from build123d import *

# Parameters (mm, degrees)
CROQUIS1_R              = 20
CROQUIS1_R_2            = 1.5
SALIENTE_EXTRUIR1_DEPTH = 2
CROQUIS2_R              = 5.75
CORTAR_EXTRUIR1_DEPTH   = 10


with BuildPart() as part:
    # Croquis1 → Saliente-Extruir1 (new body)
    with BuildSketch(Plane.XY):
        Circle(CROQUIS1_R)
        with Locations((15, 8.1)):
            Circle(CROQUIS1_R_2, mode=Mode.SUBTRACT)
        with Locations((0, -16)):
            Circle(CROQUIS1_R_2, mode=Mode.SUBTRACT)
        with Locations(Location((-15, 8.1, 0), (0, 0, 180))):
            Circle(CROQUIS1_R_2, mode=Mode.SUBTRACT)
    extrude(amount=SALIENTE_EXTRUIR1_DEPTH)

    # Croquis2 → Cortar-Extruir1 (cut)
    with BuildSketch(Plane.XY.offset(2)):
        Circle(CROQUIS2_R)
    extrude(amount=-CORTAR_EXTRUIR1_DEPTH, mode=Mode.SUBTRACT)


solid = part.part
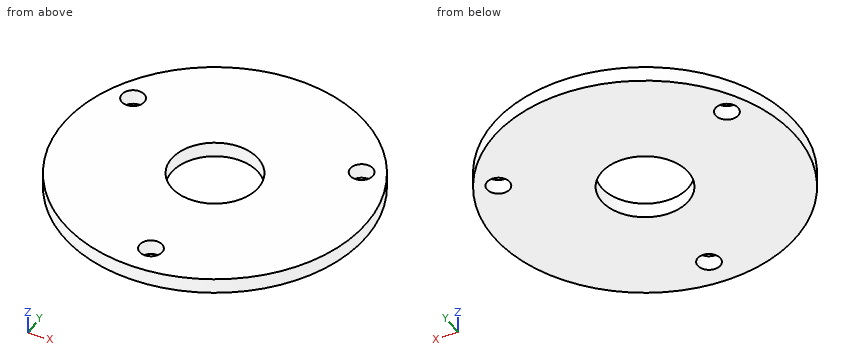
Design review of the part built by this model. Coordinates are the model's own, in mm. Coordinates: 2 decimals unless noted, no trailing zeros. Order: outer loops, then holes, each group sorted by start corner. A loop starts at its lowest first (then second) coordinate and runs counter-clockwise, first axis right, second up. Notation, with made-up numbers: (5, -4.75) - (55, -4.75) arc R20 cw to (55, 21.25) - close; hole circle Ø11 at (25, -39.5). An arc over 180 degrees is marked (long way). Put each result on its own line as item: value.
1) Take a section at D-D, the plane x = 12. Give the boundary of the cut face in (y, z).
Response values:
outline: (-16, 0) - (16, 0) - (16, 2) - (-16, 2) - close
2) Insertion check: P1, Ø13, axis at x = 0, y = 0, coming from the -Z side; P2, Ø1, axis at x = 7.5, z = 0.5, coming from the -Y side (3 decimals); P3, Ø1, axis at y = 12, z = 0.5, coming from the -X side; P4, Ø1, axis at y = -4, z = 0.5, coming from the -X side. Each pin has a flat end and moves straight along its axis. Give the tip position at first contact, or say it passes through.
Response values:
P1: stops at z = 0
P2: stops at y = -18.735
P3: stops at x = -16.36
P4: stops at x = -19.69
3) Take a section at A-A, the plane y = -16. Give the boundary of the cut face in (x, z).
Response values:
outline: (-12, 0) - (-1.5, 0) - (-1.5, 2) - (-12, 2) - close; (1.5, 0) - (12, 0) - (12, 2) - (1.5, 2) - close
4) Wall thickness on L1, parallel to Y at x = 0, z = 1.2; L2, parallel to X at y = -15.5, z = 1.55; L3, parallel to Y at x = 16, z = 0.35: over which ranges is each line inside the solid? List them lowest first. Write a range as from..to.
Response values:
L1: y = -20..-17.5, -14.5..-5.75, 5.75..20
L2: x = -12.64..-1.41, 1.41..12.64
L3: y = -12..6.98, 9.22..12
5) Take a section at B-B, the plane x = 4.5. Give the boundary of the cut face in (y, z), and give its area (3 significant figures).
Response values:
outline: (-19.49, 0) - (-3.58, 0) - (-3.58, 2) - (-19.49, 2) - close; (3.58, 0) - (19.49, 0) - (19.49, 2) - (3.58, 2) - close
area: 63.6 mm²
6) Take a section at C-C, the plane z = 1.6. Give the boundary of the cut face in (x, y), and give its area (3 significant figures).
Response values:
outline: circle Ø40 at (0, 0); hole circle Ø3 at (-15, 8.1); hole circle Ø11.5 at (0, 0); hole circle Ø3 at (0, -16); hole circle Ø3 at (15, 8.1)
area: 1,130 mm²
